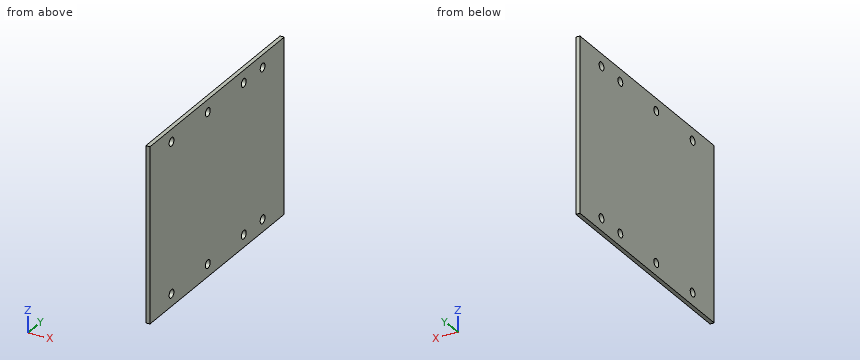
```python
from build123d import *

# Parameters (mm, degrees)
SKETCH1_W           = 133.35
SKETCH1_H           = 177.8
BOSS_EXTRUDE1_DEPTH = 3.175
SKETCH2_R           = 3.175
CUT_EXTRUDE1_DEPTH  = 112.17034789


with BuildPart() as part:
    # Sketch1 → Boss-Extrude1 (new body)
    with BuildSketch(Plane(origin=(0, 0, 0), x_dir=(0, 0, -1), z_dir=(1, 0, 0))):
        Rectangle(SKETCH1_W, SKETCH1_H)
    extrude(amount=-BOSS_EXTRUDE1_DEPTH)

    # Sketch2 → Cut-Extrude1 (cut, through all)
    with BuildSketch(Plane(origin=(0, 0, 0), x_dir=(0, 0, -1), z_dir=(1, 0, 0))):
        with Locations((-57.15, -60.325)):
            Circle(SKETCH2_R)
        with Locations((-57.15, -12.275000088)):
            Circle(SKETCH2_R)
        with Locations(Location((57.15, -12.275000088, 0), (0, 0, 180))):
            Circle(SKETCH2_R)
        with Locations(Location((57.15, -60.325, 0), (0, 0, 180))):
            Circle(SKETCH2_R)
        with Locations((-57.15, 60.325)):
            Circle(SKETCH2_R)
        with Locations((-57.15, 35.349999912)):
            Circle(SKETCH2_R)
        with Locations(Location((57.15, 35.349999912, 0), (0, 0, 180))):
            Circle(SKETCH2_R)
        with Locations(Location((57.15, 60.325, 0), (0, 0, 180))):
            Circle(SKETCH2_R)
    extrude(amount=-CUT_EXTRUDE1_DEPTH, mode=Mode.SUBTRACT)


solid = part.part
```
For this review, take the finished solid that the model builds, in its own axes (mm). Round coordinates to 2 decimals unless told otherwise and drop trailing zeros. Write each loop counter-clockwise with the first axis right and the second up, starting at its lowest first coordinate (ties: lowest second). Pieces come first, ordered by that corner, then holes. Notation, with made-up numbers: (66, 28) - (114, 28) arc R27 cw to (114, 51) - close; hole circle Ø1 at (6.25, -13). An arc over 180 degrees is marked (long way). Answer as a JSON object with one key per item and string values.
1. We need section B-B on z = 57.15. Give the boundary of the cut face in (x, y) (3 decimals), then the cut area to 3 significant figures.
Response values:
{"outline": "(-3.175, -88.9) - (0, -88.9) - (0, -63.5) - (-3.175, -63.5) - close; (-3.175, -57.15) - (0, -57.15) - (0, -15.45) - (-3.175, -15.45) - close; (-3.175, -9.1) - (0, -9.1) - (0, 32.175) - (-3.175, 32.175) - close; (-3.175, 38.525) - (0, 38.525) - (0, 57.15) - (-3.175, 57.15) - close; (-3.175, 63.5) - (0, 63.5) - (0, 88.9) - (-3.175, 88.9) - close", "area": "484 mm2"}
2. We need section A-A on y = 35.35. Give the boundary of the cut face in (x, z) (3 decimals), then the cut area to 3 significant figures.
Response values:
{"outline": "(-3.175, -66.675) - (0, -66.675) - (0, -60.325) - (-3.175, -60.325) - close; (-3.175, -53.975) - (0, -53.975) - (0, 53.975) - (-3.175, 53.975) - close; (-3.175, 60.325) - (0, 60.325) - (0, 66.675) - (-3.175, 66.675) - close", "area": "383 mm2"}
3. To check wall thickness, follow line 1 along Y through (x, z) = (-1.25, 57.15) (3 decimals); line 2 along Z through (x, y) = (-0.9, 35.35) (3 decimals); line 3 along Y through (x, z) = (-2.6, -56.5). State the ranges of each line that lie inside material, in increasing order.
Response values:
{"line 1": "y = -88.9 to -63.5, -57.15 to -15.45, -9.1 to 32.175, 38.525 to 57.15, 63.5 to 88.9", "line 2": "z = -66.675 to -60.325, -53.975 to 53.975, 60.325 to 66.675", "line 3": "y = -88.9 to -63.43, -57.22 to -15.38, -9.17 to 32.24, 38.46 to 57.22, 63.43 to 88.9"}
